from build123d import *

# Parameters (mm, degrees)
SKETCH_1_W                    = 34
SKETCH_1_H                    = 40
EXTRUDE_326_DEPTH             = 7.9
HOLE_WIZARD_40_M5_D           = 5.5
HOLE_WIZARD_40_M5_CSINK_D     = 10.4
HOLE_WIZARD_40_M5_CSINK_ANGLE = 90
HOLE_WIZARD_M3_D              = 2.5
HOLE_WIZARD_M3_CSINK_D        = 3.05
HOLE_WIZARD_M3_CSINK_ANGLE    = 90
CHAMFER_1_SIZE                = 3
SKETCH_7_W                    = 11.5
SKETCH_7_H                    = 40
EXTRUDE_40_DEPTH              = 1


with BuildPart() as part:
    # Эскиз1 → Extrude 326 (new body)
    with BuildSketch(Plane(origin=(0, 0, 0), x_dir=(1, 0, 0), z_dir=(0, 1, 0))):
        Rectangle(SKETCH_1_W, SKETCH_1_H)
    extrude(amount=EXTRUDE_326_DEPTH)

    # Крепление к профилю 40 - M5 (through all)
    with Locations(Plane(origin=(0, 7.9, 0), x_dir=(-1, 0, 0), z_dir=(0, 1, 0))):
        with Locations((0, 0)):
            CounterSinkHole(HOLE_WIZARD_40_M5_D / 2, HOLE_WIZARD_40_M5_CSINK_D / 2, counter_sink_angle=HOLE_WIZARD_40_M5_CSINK_ANGLE)

    # Крепление датчика M3 (through all)
    with Locations(Plane(origin=(0, 7.9, 0), x_dir=(-1, 0, 0), z_dir=(0, 1, 0))):
        with Locations((5.55, 8.95), (-5.55, 8.95)):
            CounterSinkHole(HOLE_WIZARD_M3_D / 2, HOLE_WIZARD_M3_CSINK_D / 2, counter_sink_angle=HOLE_WIZARD_M3_CSINK_ANGLE)

    # Фаска1
    chamfer_1_edges = [part.edges().sort_by_distance(p)[0] for p in [
        (-17, 7.9, 0),
        (17, 7.9, 0),
        (0, 7.9, -20),
    ]]
    chamfer(chamfer_1_edges, length=CHAMFER_1_SIZE)

    # Эскиз7 → Направляющая профиля 40 (add)
    with BuildSketch(Plane.XZ):
        Rectangle(SKETCH_7_W, SKETCH_7_H)
    extrude(amount=EXTRUDE_40_DEPTH)


solid = part.part
Build history of the part. All positions in model axes, mm. A direction names the side the tool comes from. Coordinates: 2 decimals unless noted, no trailing zeros. Order: outer loops, then holes, each group sorted by start corner. A loop starts at its lowest first (then second) coordinate and runs counter-clockwise, first axis right, second up. Notation, with made-up numbers: (55.25, 50.25) - (94.25, 50.25) arc R24 cw to (94.25, 81.25) - close; hole circle Ø9 at (44.5, 37). An arc over 180 degrees is marked (long way). Put each result on its own line as item: value.
1. Saw through at C-C (z = 8.95). Write the cut outline in (x, y) (3 decimals), and give its area (3 significant figures).
Answer sheet:
outline: (-17, 0) - (-6.8, 0) - (-6.8, 7.625) - (-7.075, 7.9) - (-14, 7.9) - (-17, 4.9) - close; (-5.75, -1) - (5.75, -1) - (5.75, 0) - (4.3, 0) - (4.3, 7.625) - (4.025, 7.9) - (-4.025, 7.9) - (-4.3, 7.625) - (-4.3, 0) - (-5.75, 0) - close; (6.8, 0) - (17, 0) - (17, 4.9) - (14, 7.9) - (7.075, 7.9) - (6.8, 7.625) - close
area: 231 mm^2
2. Saw through at B-B (y = 6.25). Write the cut outline in (x, z).
Answer sheet:
outline: (-15.65, -18.65) - (15.65, -18.65) - (15.65, 20) - (-15.65, 20) - close; hole circle Ø2.5 at (-5.55, 8.95); hole circle Ø7.1 at (0, 0); hole circle Ø2.5 at (5.55, 8.95)
3. Probe line 1 along X through (y, z) = (4.75, 8.95); line 2 along Z through (x, y) = (0, 4.75); line 3 along X through (y, z) = (3, 0). List the from-to ranges inside material, lowest first. Write a range as [from, to].
Answer sheet:
line 1: x = [-17, -6.8], [-4.3, 4.3], [6.8, 17]
line 2: z = [-20, -2.75], [2.75, 20]
line 3: x = [-17, -2.75], [2.75, 17]
4. Saw through at D-D (x = 0). Write the cut outline in (y, z).
Answer sheet:
outline: (-1, -20) - (4.9, -20) - (7.9, -17) - (7.9, -5.2) - (5.45, -2.75) - (0, -2.75) - (0, 2.75) - (5.45, 2.75) - (7.9, 5.2) - (7.9, 20) - (-1, 20) - close
5. Drop flat-ended pins along their axis: P1, Ø2, axis at x = 5.55, z = 8.95, coming from the +Y side; P2, Ø9, axis at x = -12.5, z = 10, coming from the -Y side; P3, Ø6, axis at x = 1, z = 0.5, coming from the +Y side. Give the stop position or say it passes through.
Answer sheet:
P1: stops at y = 0
P2: stops at y = 0
P3: stops at y = 6.82
6. Saw through at A-A (z = 0). Write the cut outline in (x, y), and give its area (3 significant figures).
Answer sheet:
outline: (-17, 0) - (-5.75, 0) - (-5.75, -1) - (5.75, -1) - (5.75, 0) - (17, 0) - (17, 4.9) - (14, 7.9) - (5.2, 7.9) - (2.75, 5.45) - (2.75, 0) - (-2.75, 0) - (-2.75, 5.45) - (-5.2, 7.9) - (-14, 7.9) - (-17, 4.9) - close
area: 222 mm^2
7. Pull direction Z, two halves, no side cores. Call faces 4 (the face through (11, 0, 0)), 5 (the face through (0, 2, -20)), 6 (the face through (-2.277, 5.569, -1.746)): pulls with the +Z half, pulls with the -Z half, needs draft (parallel to the pull), parting line crosses it, or undercut.
Answer sheet:
face 4: needs draft
face 5: pulls with the -Z half
face 6: undercut
8. Tool access for faces 1 (the face through (-5, 0, 9)), 2 (the face through (-0.2, 7.9, 5.4)), 3 (the face through (-11, 0, 0)): list every direction of +Z, -Z, +X, -X, +Y, -Y with a clear straight run to the whole face (end or side of a thin tool).
Answer sheet:
face 1: +Y
face 2: +Z, -Z, +X, -X, +Y
face 3: +Z, -Z, -X, -Y
